Autodesk Fusion 360 part; units mm, degrees
sketch "Sketch1" plane through (0, 0, 0) normal (0, 0, 1) x (1, 0, 0)
  circle A0 centre (0, 0) radius 4.1
  circle A1 centre (0, 0) radius 35
  circle A2 centre (0, 0) radius 8 construction
  circle A3 centre (0, 0) radius 25 construction
  circle A4 centre (0, 25) radius 6.3
  circle A5 centre (0, 25) radius 3.2
  circle A6 centre (0, 8) radius 1.6
  circle A7 centre (-6.9282, -4) radius 1.6
  circle A8 centre (6.9282, -4) radius 1.6
  circle A9 centre (-17.6777, 17.6777) radius 3.2
  circle A10 centre (-25, 0) radius 3.2
  circle A11 centre (-17.6777, -17.6777) radius 3.2
  circle A12 centre (0, -25) radius 3.2
  circle A13 centre (17.6777, -17.6777) radius 3.2
  circle A14 centre (25, 0) radius 3.2
  circle A15 centre (17.6777, 17.6777) radius 3.2
  dimension "d1" = 8.2
  dimension "d2" = 50
  dimension "d3" = 70
  dimension "d4" = 16
  dimension "d5" = 12.6
  dimension "d6" = 6.4
  dimension "d7" = 3.2
  dimension "d9" = 360
  dimension "d11" = 360
extrude "Extrude1" add sketch "Sketch1" along normal blind 6 contours A1 | A4
Source: CAD feature listing. Evaluate the final solid. Frame: model axes, mm. Coordinates: 2 decimals unless noted, no trailing zeros. Loops run counter-clockwise (first coordinate to the right, second up) from the corner with the lowest first, then second, coordinate; pieces in that order, holes last. Notation, with made-up numbers: M 47,1.25 L 53,1.25 A20 ccw 53,33.25 Z; hole C -9,-31.5 d11. An arc over 180 degrees is marked long. Use CSV: the item, a comma, the result in double quotes.
(1) Cut plane A-A on y = 0. Return loops of the section in (x, z), and give its area (3 significant figures).
Answers follow:
outline,"M -35,0 L -28.2,0 L -28.2,6 L -35,6 Z; M -21.8,0 L -4.1,0 L -4.1,6 L -21.8,6 Z; M 4.1,0 L 21.8,0 L 21.8,6 L 4.1,6 Z; M 28.2,0 L 35,0 L 35,6 L 28.2,6 Z"
area,"294 mm²"
(2) Line query: line 1 (Y direction, x = 0, z = 2.7); line 2 (Y direction, x = -15, z = 0.3); line 3 (Y direction, x = 20, z = 4.9). Output: solid intervals per line, ascending. Write a range as [from, to].
Answers follow:
line 1,"[-35, -28.2], [-21.8, -4.1], [4.1, 6.4], [9.6, 21.8], [28.2, 35]"
line 2,"[-31.62, -19.43], [-15.93, 15.93], [19.43, 31.62]"
line 3,"[-28.72, -19.88], [-15.48, 15.48], [19.88, 28.72]"
(3) Cut plane B-B on y = -23. Return loops of the section in (x, z), and give its area (3 significant figures).
Answers follow:
outline,"M -26.38,0 L -2.5,0 L -2.5,6 L -26.38,6 Z; M 2.5,0 L 26.38,0 L 26.38,6 L 2.5,6 Z"
area,"287 mm²"
(4) Contact query for flat-ended pins moving along their axis: pin 1 (3 mm diameter, centred on x = 12, z = 0.5, fed in from -Y); pin 2 (2 mm diameter, centred on y = -4, z = 1, fed in from +X); pin 3 (2 mm diameter, centred on y = 16.5, z = 2.5, fed in from -X). Output: stop coordinate, or through.
Answers follow:
pin 1,"y = -33.39"
pin 2,"x = 34.87"
pin 3,"x = -31.38"
(5) Draft query along X for faces 1 (the face through (-28, 21, 3)), 2 (the face through (0, -7, 6)), 3 (the face through (-7.28, -2.44, 2.96)). Return one class per face: pulls with the +X half, pulls with the -X half, needs draft (parallel to the pull), parting line crosses it, or undercut.
Answers follow:
face 1,"parting line crosses it"
face 2,"needs draft"
face 3,"undercut"
(6) Cut plane C-C on x = -0.5. Return loops of the section in (y, z).
Answers follow:
outline,"M -35,0 L -28.16,0 L -28.16,6 L -35,6 Z; M -21.84,0 L -4.07,0 L -4.07,6 L -21.84,6 Z; M 4.07,0 L 6.48,0 L 6.48,6 L 4.07,6 Z; M 9.52,0 L 21.84,0 L 21.84,6 L 9.52,6 Z; M 28.16,0 L 35,0 L 35,6 L 28.16,6 Z"
(7) Cut plane D-D on z = 3.1. Give the number of separate pieces and of enclosed holes in the cut face, and give its area (3 significant figures).
Answers follow:
separate pieces,"1"
enclosed holes,"12"
area,"3,510 mm²"
